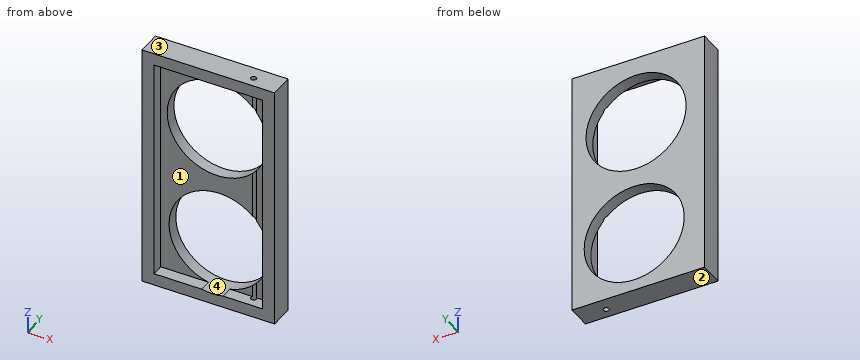
from build123d import *

# Parameters (mm, degrees)
F0_W     = 84.156403
F0_H     = 156.948597
F1_DEPTH = 15.24
F2_T     = -7.62
F4_D     = 63.5
F6_D     = 63.5
F8_D     = 3.5


with BuildPart() as f1:
    # F0 (on Front) → F1 (new body)
    with BuildSketch(Plane.XZ):
        with Locations((-25.185494, 2.457119)):
            Rectangle(F0_W, F0_H)
    extrude(amount=F1_DEPTH)

    # F2
    f2_openings = [f1.faces().sort_by_distance(p)[0] for p in [
        (-25.185495, -15.24, 2.45712),
    ]]
    offset(amount=F2_T, openings=f2_openings)

    # F4 (through all)
    with Locations(Plane(origin=(0, 0, 0), x_dir=(-1, 0, 0), z_dir=(0, 1, 0))):
        with Locations((23.760062, 37.687458)):
            Hole(F4_D / 2)

    # F6 (through all)
    with Locations(Plane(origin=(0, 0, 0), x_dir=(-1, 0, 0), z_dir=(0, 1, 0))):
        with Locations((22.599144, -37.385169)):
            Hole(F6_D / 2)

    # F8 (through all)
    with Locations(Plane(origin=(0, 0, -76.017179), x_dir=(1, 0, 0), z_dir=(0, 0, -1))):
        with Locations((0, 8.793092)):
            Hole(F8_D / 2)


solid = f1.part
For this review, take the finished solid that the model builds, in its own axes (mm). Face numbers are marked on the shaded views. A direction names the side the tool comes from. Round coordinates to 2 decimals unless told otherwise and drop trailing zeros. Order: outer loops, then holes, each group sorted by start corner. A loop starts at its lowest first (then second) coordinate and runs counter-clockwise, first axis right, second up. Notation, with made-up numbers: M -23,-34 L -9,-34 A26 ccw -9,-2 Z; hole C 85,-1.75 d5. An arc over 180 degrees is marked long. Use a Markdown table: item, result. Add a question column.
Item 1: Add section A-A, the plane y = -13.5. Give the boundary of the cut face in (x, z), then the cut area to 3 significant figures.
Item 2: Add section C-C, the plane x = -5. Give the boundary of the cut face in (y, z), then the cut area to 3 significant figures.
Item 3: Insertion check: pin 1 (3 mm diameter, centred on x = 0, y = -8.79, fed in from -Z); pin 2 (12 mm diameter, centred on x = -29.5, z = 9.5, fed in from +Y); pin 3 (3.5 mm diameter, centred on x = -9.5, z = -65.5, fed in from -Y). Each pin has a flat end and moves straight along its axis. Give the tip position at first contact, or say it passes through.
Item 4: Tool access review of the marked faces 1 and 2: name each direction out of +Z, -Z, +X, -X, +Y, -Y from which nothing blocks a thin tool from reaching the whole face with its end or side.
Item 5: Add section B-B, the plane z = 40.5. Give the boundary of the cut face in (x, y).
Item 6: To check wall thickness, follow line 1 along Z through (x, y) = (-3, -10.5); line 2 along X through (y, z) = (-11.25, 27); line 3 along Z through (x, y) = (-19, -2). State the ranges of each line that lie inside material, in increasing order.
Item 7: Mouldability with a two-part tool opening along X and no side actions: class the marked faces 3 and 4 as released by +X, released by -X, zero draft, split by the parting line, or undercut.
Item 8: Add section D-D, the plane y = -4.25. Give the boundary of the cut face in (x, z).
Geometry results:
| question | item | result |
|---|---|---|
| 1 | outline | M -67.26,-76.02 L 16.89,-76.02 L 16.89,80.93 L -67.26,80.93 Z; hole M -59.64,-68.4 L -29.4,-68.4 A31.75 ccw -15.79,-68.4 L 9.27,-68.4 L 9.27,73.31 L -59.64,73.31 Z |
| 1 | area | 3,440 mm² |
| 2 | outline | M -15.24,-76.02 L 0,-76.02 L 0,-63.81 L -7.62,-63.81 L -7.62,-68.4 L -15.24,-68.4 Z; M -15.24,73.31 L -7.62,73.31 L -7.62,63.3 L 0,63.3 L 0,80.93 L -15.24,80.93 Z; M -7.62,-10.96 L 0,-10.96 L 0,12.07 L -7.62,12.07 Z |
| 2 | area | 519 mm² |
| 3 | pin 1 | passes through |
| 3 | pin 2 | stops at y = 0 |
| 3 | pin 3 | stops at y = -7.62 |
| 4 | face 1 | -Y |
| 4 | face 2 | -Z, +X, -X, +Y, -Y |
| 5 | outline | M -67.26,-15.24 L -59.64,-15.24 L -59.64,-7.62 L -55.39,-7.62 L -55.39,0 L -67.26,0 Z; M 7.87,-7.62 L 9.27,-7.62 L 9.27,-15.24 L 16.89,-15.24 L 16.89,0 L 7.87,0 Z |
| 6 | line 1 | z = -76.02 to -68.4, 73.31 to 80.93 |
| 6 | line 2 | x = -67.26 to -59.64, 9.27 to 16.89 |
| 6 | line 3 | z = -76.02 to -68.93, -5.84 to 6.3, 69.08 to 80.93 |
| 7 | face 3 | zero draft |
| 7 | face 4 | undercut |
| 8 | outline | M -67.26,-76.02 L 16.89,-76.02 L 16.89,80.93 L -67.26,80.93 Z; hole C -23.76,37.69 d63.5; hole C -22.6,-37.39 d63.5 |
